The listing builds one solid part. Answer for the finished solid, in the listing's coordinates (mm). Face numbers are marked on the shaded views. A direction names the side the tool comes from. Give positions to 0.01 mm unless a question says otherwise; leave off trailing zeros. Write each loop counter-clockwise with the first axis right and the second up, starting at its lowest first coordinate (ties: lowest second). Pieces come first, ordered by that corner, then holes. Notation, with made-up numbers: (-8.75, 87) - (40.25, 87) arc R15 cw to (40.25, 100) - close; hole circle Ø6 at (57.25, 74). An arc over 180 degrees is marked (long way). Write each question's results on one line, items separated by ' | '. Start each with the question number.
Q1. For the marked faces 5, 6, 7 and 8, determine the directions among +Z, -Z, +X, -X, +Y, -Y from which every point of the face is accessible in a straight line to the end or side of a thin tool.
Q2. Find the intervals of material crossed by probe 1 along Y at (x, z) = (30, -19); probe 2 along Y at (x, z) = (17, 2.75); probe 3 along Z at (x, y) = (-14, 16.5), in increasing order.
Q3. Section C-C (z = 2.5) is taken. Determine the outline of the cut face in (x, y).
Q4. Section A-A (z = 23) is taken. Determine the outline of the cut face in (x, y).
Q5. Section B-B (y = 17) is taken. Determine the outline of the cut face in (x, z).
Q6. Section D-D (z = -23) is taken. State how many separate pieces and enclosed holes the cut face has, plus the area to 3 significant figures.
Q7. For a pull along Y with two mould halves and no side action, classify the marked faces 1, 2, 3 and 4 as pulls with the +Y half, pulls with the -Y half, needs draft (parallel to the pull), parting line crosses it, or undercut.
Q8. Flat-ended cylindrical pins translate along their axes: pin 1 Ø9.5 at (x, z) = (-18, -23) entering from -Y; pin 2 Ø4 at (x, y) = (-16, -57.5) entering from -Z; pin 3 Ø12 at (x, y) = (2.5, -14.5) entering from +Z; pin 4 Ø5.5 at (y, z) = (-56.5, -21.5) entering from +X. Find the tip coordinate at first contact, or state that the pin passes through.
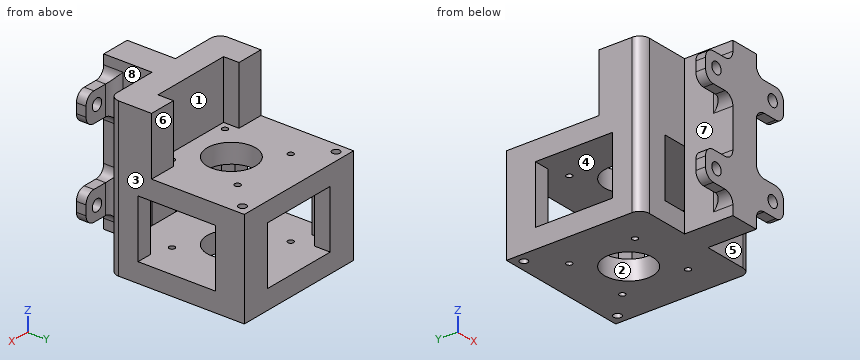
```python
from build123d import *

# Parameters (mm, degrees)
SKETCH1_W                 = 70
SKETCH1_H                 = 70
SKETCH1_R                 = 12.5
SKETCH1_R_2               = 1.5
BOSS_EXTRUDE1_DEPTH       = 10
BOSS_EXTRUDE2_DEPTH       = 30
BOSS_EXTRUDE3_DEPTH       = 30
CIRPATTERN1_COUNT         = 4
SKETCH4_R                 = 2
CUT_EXTRUDE1_DEPTH        = 50
SKETCH6_W                 = 15
SKETCH6_H                 = 80
BOSS_EXTRUDE4_DEPTH       = 25
SKETCH7_W                 = 50
SKETCH7_H                 = 15
BOSS_EXTRUDE5_DEPTH       = 5
F_6_0MM_DOWEL_HOLE1_D     = 6
F_6_0MM_DOWEL_HOLE1_DEPTH = 5
FILLET1_R                 = 5
FILLET2_R                 = 5
FILLET3_R                 = 5


with BuildPart() as part:
    # Sketch1 → Boss-Extrude1 (new body)
    with BuildSketch(Plane.XY):
        Rectangle(SKETCH1_W, SKETCH1_H)
        Circle(SKETCH1_R, mode=Mode.SUBTRACT)
        with Locations((17, 17)):
            Circle(SKETCH1_R_2, mode=Mode.SUBTRACT)
        with Locations((-17, 17)):
            Circle(SKETCH1_R_2, mode=Mode.SUBTRACT)
        with Locations((17, -17)):
            Circle(SKETCH1_R_2, mode=Mode.SUBTRACT)
        with Locations((-17, -17)):
            Circle(SKETCH1_R_2, mode=Mode.SUBTRACT)
    boss_extrude1 = extrude(amount=BOSS_EXTRUDE1_DEPTH)

    # Sketch2 → Boss-Extrude2 (add)
    with BuildSketch(Plane.XY.offset(10)):
        Polygon((-21, -13), (-21, -21), (21, -21), (21, -13), (35, -13), (35, -35), (-35, -35), (-35, -13), align=None)
    extrude(amount=BOSS_EXTRUDE2_DEPTH)

    # Sketch3 → Boss-Extrude3 (add)
    with BuildSketch(Plane(origin=(0, 0, 0), x_dir=(-1, 0, 0), z_dir=(0, 0, -1))):
        Polygon((27, 20), (35, 20), (35, 35), (20, 35), (20, 27), (27, 27), align=None)
    boss_extrude3 = extrude(amount=BOSS_EXTRUDE3_DEPTH)

    # CirPattern1: Boss-Extrude3 ×4 about axis
    cirpattern1_axis = Axis((0, 0, 0), (0, 0, 1))
    for i in range(1, CIRPATTERN1_COUNT):
        add(boss_extrude3.rotate(cirpattern1_axis, i * 360 / CIRPATTERN1_COUNT))

    # Mirror1: Boss-Extrude1 across plane
    add(boss_extrude1.mirror(Plane(origin=(0, 0, -15), x_dir=(1, 0, 0), z_dir=(0, 0, -1))))

    # Sketch4 → Cut-Extrude1 (cut)
    with BuildSketch(Plane(origin=(0, 0, -40), x_dir=(-1, 0, 0), z_dir=(0, 0, -1))):
        with Locations((30, 30)):
            Circle(SKETCH4_R)
    cut_extrude1 = extrude(amount=-CUT_EXTRUDE1_DEPTH, mode=Mode.SUBTRACT)

    # Mirror2: Cut-Extrude1 across plane
    add(cut_extrude1.mirror(Plane(origin=(0, 0, 0), x_dir=(0, 0, 1), z_dir=(1, 0, 0))), mode=Mode.SUBTRACT)

    # Sketch6 → Boss-Extrude4 (add)
    with BuildSketch(Plane.XZ.offset(35)):
        Rectangle(SKETCH6_W, SKETCH6_H)
    extrude(amount=BOSS_EXTRUDE4_DEPTH)

    # Sketch7 → Boss-Extrude5 (add)
    with BuildSketch(Plane.XZ.offset(60)):
        with Locations((0, 22.5)):
            Rectangle(SKETCH7_W, SKETCH7_H)
        with Locations((0, -22.5)):
            Rectangle(SKETCH7_W, SKETCH7_H)
    extrude(amount=-BOSS_EXTRUDE5_DEPTH)

    # Ø6.0mm Dowel Hole1
    with Locations(Plane(origin=(-18, -60, 23), x_dir=(0, 0, -1), z_dir=(0, -1, 0))):
        with Locations((0, 0), (0, 36), (46, 0), (46, 36)):
            Hole(F_6_0MM_DOWEL_HOLE1_D / 2, depth=F_6_0MM_DOWEL_HOLE1_DEPTH)

    # Fillet1
    fillet1_edges = [part.edges().sort_by_distance(p)[0] for p in [
        (25, -57.5, 15),
        (-25, -57.5, 30),
        (25, -57.5, 30),
        (7.5, -57.5, 15),
        (-7.5, -57.5, 15),
        (-25, -57.5, 15),
        (7.5, -57.5, 30),
        (-7.5, -57.5, 30),
        (25, -57.5, -30),
        (-25, -57.5, -15),
        (25, -57.5, -15),
        (7.5, -57.5, -30),
        (-7.5, -57.5, -30),
        (-25, -57.5, -30),
        (7.5, -57.5, -15),
        (-7.5, -57.5, -15),
    ]]
    fillet(fillet1_edges, radius=FILLET1_R)

    # Fillet2
    fillet2_edges = [part.edges().sort_by_distance(p)[0] for p in [
        (-7.5, -55, 22.5),
        (-7.5, -55, -22.5),
        (7.5, -55, -22.5),
        (7.5, -55, 22.5),
    ]]
    fillet(fillet2_edges, radius=FILLET2_R)

    # Fillet3
    fillet3_edges = [part.edges().sort_by_distance(p)[0] for p in [
        (-35, -35, 0),
        (35, -35, 0),
    ]]
    fillet(fillet3_edges, radius=FILLET3_R)


solid = part.part
```
Answers below:
1) face 5: +Z, -Z, +X | face 6: +Z, +X, -X, +Y | face 7: -X | face 8: +X
2) probe 1: y = -35 to -20, 20 to 28, 32 to 35 | probe 2: y = -35 to -18.5, -15.5 to 15.5, 18.5 to 35 | probe 3: z = -40 to -30, 0 to 10
3) outline: (-35, -30) arc R5 ccw to (-30, -35) - (-7.5, -35) - (-7.5, -60) - (7.5, -60) - (7.5, -35) - (30, -35) arc R5 ccw to (35, -30) - (35, 35) - (-35, 35) - close; hole circle Ø4 at (-30, 30); hole circle Ø3 at (-17, -17); hole circle Ø3 at (-17, 17); hole circle Ø25 at (0, 0); hole circle Ø3 at (17, -17); hole circle Ø3 at (17, 17); hole circle Ø4 at (30, 30)
4) outline: (-35, -30) arc R5 ccw to (-30, -35) - (-7.5, -35) - (-7.5, -50) arc R5 cw to (-12.5, -55) - (-15, -55) - (-15, -60) - (15, -60) - (15, -55) - (12.5, -55) arc R5 cw to (7.5, -50) - (7.5, -35) - (30, -35) arc R5 ccw to (35, -30) - (35, -13) - (21, -13) - (21, -21) - (-21, -21) - (-21, -13) - (-35, -13) - close; (-25, -60) - (-21, -60) - (-21, -55) - (-25, -55) - close; (21, -60) - (25, -60) - (25, -55) - (21, -55) - close
5) outline: (-35, -40) - (-18.5, -40) - (-18.5, -30) - (-35, -30) - close; (-35, 0) - (-18.5, 0) - (-18.5, 10) - (-35, 10) - close; (-15.5, -40) - (15.5, -40) - (15.5, -30) - (-15.5, -30) - close; (-15.5, 0) - (15.5, 0) - (15.5, 10) - (-15.5, 10) - close; (18.5, -40) - (35, -40) - (35, -30) - (18.5, -30) - close; (18.5, 0) - (35, 0) - (35, 10) - (18.5, 10) - close
6) separate pieces: 7 | enclosed holes: 2 | area: 1,170 mm2
7) face 1: pulls with the +Y half | face 2: undercut | face 3: needs draft | face 4: undercut
8) pin 1: stops at y = -60 | pin 2: stops at z = -30 | pin 3: stops at z = 10 | pin 4: stops at x = 25
